Could you check a few things on this model? Use its own coordinates, in mm. A direction names the side the tool comes from. Round coordinates to 2 decimals unless told otherwise and drop trailing zeros. Loops run counter-clockwise (first coordinate to the right, second up) from the corner with the lowest first, then second, coordinate; pieces in that order, holes last. Notation, with made-up numbers: (22.5, 14.25) -> (65.5, 14.25) arc R19 ccw to (65.5, 25.25) -> close; hole circle Ø2 at (-27, -21.75). An arc over 180 degrees is marked (long way). Write each question's results on one line, items separated by ' | '. Start each with the question number.
1) Imagine slicing it at D-D, the plane y = -15.5. List the corners of the cut face in (x, z) for me.
2) If I drill on probe 1 along Y at (x, z) = (0, 11.65); probe 2 along Z at (x, y) = (21, -11); probe 3 along Y at (x, z) = (1.5, 4.75), over which ranges is the centre line in solid material (lowest first)?
3) Imagine slicing it at A-A, the plane y = 0. List the corners of the cut face in (x, z) for me, plus the area to 3 significant figures.
4) For P1, Ø4, axis at x = -1, y = 0.5, coming from the -Z side; P2, Ø5, axis at x = -10.5, z = 10, coming from the +Y side; P3, Ø1.5, axis at x = 9.5, z = 9, coming from the +Y side; P4, Ø4, axis at x = 0, y = 0, coming from the -Z side, each with a flat end and sliding along its axis, tell me the tip position at first contact or that it passes through.
5) Which directions (+Z, -Z, +X, -X, +Y, -Y) give clear straight access to the entire face, cutting with the end or side of a thin tool? Please do faces 1 (the cylindrical face through (4.38, 8.43, 10.47)), 2 (the flat face through (0, 3, 10.5)), 3 (the flat face through (0, -6, 0)).
6) We'd pull the mould along X, two halves only. Please class faces 4 (the cylindrical face through (3.746, 0.165, 5.176)), 5 (the flat face through (0, -12, 8.5)), 6 (the cylindrical face through (-5.961, 26.846, 4.19)): pulls with the +X half, pulls with the -X half, needs draft (parallel to the pull), parting line crosses it, or undercut.
7) Imagine slicing it at C-C, the plane z = 7.5. List the corners of the cut face in (x, y) for me.
Autodesk Inventor part; units mm, degrees
ref_plane "YZ Plane" through (0, 0, 0) normal (1, 0, 0) x (0, 1, 0)
ref_plane "XZ Plane" through (0, 0, 0) normal (0, 1, 0) x (-1, 0, 0)
ref_plane "XY Plane" through (0, 0, 0) normal (0, 0, 1) x (1, 0, 0)
sketch "Boceto1" plane through (0, 0, 0) normal (0, 0, 1) x (1, 0, 0)
  circle A0 centre (0, 0) radius 27.5
  circle A1 centre (0, 0) radius 2.5
  dimension "d0" = 55
  dimension "d3" = 5
extrude "Extrusión1" add sketch "Boceto1" along normal blind 8.5
sketch "Boceto2" plane through (0, 0, 8.5) normal (0, 0, 1) x (1, 0, 0)
  circle A0 centre (0, 0) radius 2.5
  circle A1 centre (0, 0) radius 9.5
  dimension "d4" = 19
extrude "Extrusión2" add sketch "Boceto2" along normal blind 4
sketch "Boceto3" plane through (0, 0, 0) normal (0, 0, -1) x (-1, 0, 0)
  circle A0 centre (0, 0) radius 2.5
  circle A1 centre (0, 0) radius 3.75
  dimension "d7" = 7.5
extrude "Extrusión3" cut sketch "Boceto3" against normal blind 10.5 contours A0 | A1
properties part number "omniwheel"
Checked values:
1) outline: (-22.72, 0) -> (22.72, 0) -> (22.72, 8.5) -> (-22.72, 8.5) -> close
2) probe 1: -9.5 to -2.5, 2.5 to 9.5 | probe 2: 0 to 8.5 | probe 3: -27.46 to -3.44, 3.44 to 27.46
3) outline: (-27.5, 0) -> (-3.75, 0) -> (-3.75, 10.5) -> (-2.5, 10.5) -> (-2.5, 12.5) -> (-9.5, 12.5) -> (-9.5, 8.5) -> (-27.5, 8.5) -> close; (2.5, 10.5) -> (3.75, 10.5) -> (3.75, 0) -> (27.5, 0) -> (27.5, 8.5) -> (9.5, 8.5) -> (9.5, 12.5) -> (2.5, 12.5) -> close | area: 455 mm^2
4) P1: z = 10.5 | P2: y = 26.15 | P3: y = 26.01 | P4: through
5) face 1: +Z | face 2: -Z | face 3: -Z, +X, -X, +Y, -Y
6) face 4: undercut | face 5: needs draft | face 6: parting line crosses it
7) outline: circle Ø55 at (0, 0); hole circle Ø7.5 at (0, 0)
